```python
from build123d import *

# Parameters (mm, degrees)
F0_R     = 50
F0_R_2   = 47.5
F1_DEPTH = 5
F3_DEPTH = 2


# Not quite as in the source:
# - a fillet or chamfer that OpenCascade refuses, or shapes differently, is made with other operations: its cross-section is extruded or revolved along the edge and cut away or added


with BuildPart() as f1:
    # F0 (on Top) → F1 (new body)
    with BuildSketch(Plane.XY):
        Circle(F0_R)
        Circle(F0_R_2, mode=Mode.SUBTRACT)
    extrude(amount=F1_DEPTH)

    # F2: fillet of radius 5 on 1 edges, made by hand

    # F2_s1 → F2_t2 (revolve, cut)
    with BuildSketch(Plane.XZ):
        with BuildLine():
            ThreePointArc((50, 0.6698729811), (49.3301270189, 3.1698729811), (47.5, 5))
            Line((47.5, 5), (50, 5))
            Line((50, 5), (50, 0.6698729811))
        make_face()
    revolve(axis=Axis((0, 0, 5), (0, 0, 1)), mode=Mode.SUBTRACT)

    # F0 (on Top) → F3 (join)
    with BuildSketch(Plane.XY):
        Circle(F0_R_2)
    extrude(amount=F3_DEPTH)


solid = f1.part
```
Could you check a few things on this model? Use its own coordinates, in mm. Round coordinates to 2 decimals unless told otherwise and drop trailing zeros. Write each loop counter-clockwise with the first axis right and the second up, starting at its lowest first coordinate (ties: lowest second). Pieces come first, ordered by that corner, then holes.
(1) Suppose I cut it at C-C on z = 4.1. Write out the boundary of the cut face in (x, y).
Findings below:
outline: circle Ø97.28 at (0, 0); hole circle Ø95 at (0, 0)
(2) For pin 1 (1 mm diameter, centred on x = -31.5, y = -9.5, fed in from -Z); pin 2 (2 mm diameter, centred on x = -23.5, z = 2.5, fed in from -Y); pin 3 (1.5 mm diameter, centred on y = -4.5, z = 2.5, fed in from +X); pin 4 (1.5 mm diameter, centred on y = -1.5, z = 2.5, fed in from +X), each with a flat end and sliding along its axis, tell me the tip position at first contact or that it passes through.
Findings below:
pin 1: stops at z = 0
pin 2: stops at y = -44.38
pin 3: stops at x = 49.69
pin 4: stops at x = 49.86
(3) Thinking about a two-plate mould opening in X: for faces 1 (the face through (-1, 1, 2)), 2 (the face through (-1, 1, 0)), 3 (the face through (47.69, 15.02, 0.33)), which applies, +X half, -X half, draft (parallel to the pull), parting line (faces both ways), or undercut?
Findings below:
face 1: undercut
face 2: draft
face 3: parting line
(4) If I drill on probe 1 along Z at (x, y) = (-3.5, -13); probe 2 along X at (y, z) = (12, 2.3); probe 3 along X at (y, z) = (-17, 3.85), over which ranges is the centre line in solid material (lowest first)?
Findings below:
probe 1: z = 0 to 2
probe 2: x = -48.26 to -45.96, 45.96 to 48.26
probe 3: x = -45.81 to -44.35, 44.35 to 45.81
(5) Suppose I cut it at A-A on y = 0. Write out the boundary of the cut face in (x, z).
Findings below:
outline: (-50, 0) - (50, 0) - (50, 0.67) arc R5 ccw to (47.5, 5) - (47.5, 2) - (-47.5, 2) - (-47.5, 5) arc R5 ccw to (-50, 0.67) - close
